Could you check a few things on this model? Use its own coordinates, in mm. A direction names the side the tool comes from. Round coordinates to 2 decimals unless told otherwise and drop trailing zeros. Order: outer loops, then holes, each group sorted by start corner. A loop starts at its lowest first (then second) coordinate and runs counter-clockwise, first axis right, second up. Notation, with made-up numbers: (-12.75, 38) - (24.25, 38) arc R25 cw to (24.25, 70) - close; hole circle Ø4 at (72, 78). An arc over 180 degrees is marked (long way). Use one line per item in the form item = value.
from build123d import *

# Parameters (mm, degrees)
BOSS_EXTRU_1_DEPTH                  = 3.175
ESQUISSE3_W                         = 42
ESQUISSE3_H                         = 16
BOSS_EXTRU_2_DEPTH                  = 45
ESQUISSE4_W                         = 20
ESQUISSE4_H                         = 16
ENL_V_MAT_EXTRU_1_DEPTH             = 123.60232716
ESQUISSE5_W                         = 22
ESQUISSE5_H                         = 31.825
ENL_V_MAT_EXTRU_2_DEPTH             = 128.730184373
CONG_1_R                            = 5
D_GAGEMENT_M3_51_D                  = 3.9
D_GAGEMENT_M31_D                    = 3.4
ESQUISSE11_R                        = 17.225
ENL_V_MAT_EXTRU_3_DEPTH             = 123.60232716
DIAM_TRE_DU_PER_AGE_4_5_4_5_2_D     = 4.5
DIAM_TRE_DU_PER_AGE_4_5_4_5_2_DEPTH = 5.8
ENL_V_MAT_EXTRU_4_DEPTH             = 18


with BuildPart() as part:
    # Esquisse1 → Boss.-Extru.1 (new, symmetric)
    with BuildSketch(Plane(origin=(0, 0, 0), x_dir=(1, 0, 0), z_dir=(0, 1, 0))):
        with BuildLine():
            Line((-40, 59), (40, 59))
            ThreePointArc((40, 59), (99, 0), (40, -59))
            Line((40, -59), (-40, -59))
            ThreePointArc((-40, -59), (-99, 0), (-40, 59))
        make_face()
    extrude(amount=BOSS_EXTRU_1_DEPTH, both=True)

    # Esquisse3 → Boss.-Extru.2 (add)
    with BuildSketch(Plane(origin=(0, 0, 0), x_dir=(1, 0, 0), z_dir=(0, 1, 0))):
        with Locations((-62.5, 0)):
            Rectangle(ESQUISSE3_W, ESQUISSE3_H)
    extrude(amount=BOSS_EXTRU_2_DEPTH)

    # Esquisse4 → Enlèv. mat.-Extru.1 (cut, through all)
    with BuildSketch(Plane(origin=(0, 3.175, 0), x_dir=(1, 0, 0), z_dir=(0, 1, 0))):
        with Locations((-31.5, 0)):
            Rectangle(ESQUISSE4_W, ESQUISSE4_H)
    extrude(amount=-ENL_V_MAT_EXTRU_1_DEPTH, mode=Mode.SUBTRACT)

    # Esquisse5 → Enlèv. mat.-Extru.2 (cut, through all)
    with BuildSketch(Plane.XY.offset(8)):
        with Locations((-72.5, 29.0875)):
            Rectangle(ESQUISSE5_W, ESQUISSE5_H)
    extrude(amount=-ENL_V_MAT_EXTRU_2_DEPTH, mode=Mode.SUBTRACT)

    # Congé1
    cong_1_edges = [part.edges().sort_by_distance(p)[0] for p in [
        (-72.5, 13.175, -8),
        (-61.5, 13.175, 0),
        (-83.5, 13.175, 0),
        (-61.5, 29.0875, 8),
        (-61.5, 29.0875, -8),
        (-72.5, 13.175, 8),
    ]]
    fillet(cong_1_edges, radius=CONG_1_R)

    # Dégagement M3.51 (through all)
    with Locations(Plane(origin=(-41.5, 0, 0), x_dir=(0, 0, -1), z_dir=(1, 0, 0))):
        with Locations((0, 32.55)):
            Hole(D_GAGEMENT_M3_51_D / 2)

    # Dégagement M31 (through all)
    with Locations(Plane(origin=(0, 3.175, 0), x_dir=(1, 0, 0), z_dir=(0, 1, 0))):
        with Locations((60.016012145, -11.55625), (40, 23.1125), (19.983987855, -11.55625)):
            Hole(D_GAGEMENT_M31_D / 2)

    # Esquisse11 → Enlèv. mat.-Extru.3 (cut, through all)
    with BuildSketch(Plane(origin=(0, 3.175, 0), x_dir=(1, 0, 0), z_dir=(0, 1, 0))):
        with Locations(Location((40, 0, 0), (0, 0, 270))):
            Circle(ESQUISSE11_R)
    extrude(amount=-ENL_V_MAT_EXTRU_3_DEPTH, mode=Mode.SUBTRACT)

    # Diamètre du perçage Ø4.5 (4.5)2
    with Locations(Plane(origin=(0, -3.175, 0), x_dir=(-1, 0, 0), z_dir=(0, -1, 0))):
        with Locations((78.5, 0), (66.5, 0)):
            Hole(DIAM_TRE_DU_PER_AGE_4_5_4_5_2_D / 2, depth=DIAM_TRE_DU_PER_AGE_4_5_4_5_2_DEPTH)

    # Esquisse14 → Enlèv. mat.-Extru.4 (cut)
    with BuildSketch(Plane.ZY.offset(61.5)):
        Polygon((4.67653718, 32.55), (2.33826859, 36.6), (-2.33826859, 36.6), (-4.67653718, 32.55), (-2.33826859, 28.5), (2.33826859, 28.5), align=None)
    extrude(amount=-ENL_V_MAT_EXTRU_4_DEPTH, mode=Mode.SUBTRACT)


solid = part.part
Item 1: If we mould it in two halves opening along Z, with no side actions, what happens to faces 4 (the face through (-1, 0, -59)), 5 (the face through (-98.986, 0.044, 1.297)), 6 (the face through (-43.5, 34.4, 1)), 7 (the face through (-73, 13.175, 0))? For each: released by +Z, released by -Z, zero draft, split by the parting line, or undercut.
Found:
face_4 = released by -Z
face_5 = split by the parting line
face_6 = undercut
face_7 = zero draft
Item 2: I need wall thicknesses on L1, parallel to Y at x = -42.3, z = 0 (3 decimals); L2, parallel to X at y = 0, z = 10 (3 decimals); L3, parallel to Y at x = 11, z = 42.5 (3 decimals). Which ranges of each line are inside material? Lowest first, please.
Found:
L1 = -3.175 to 30.6, 34.5 to 45
L2 = -98.146 to 19.3, 20.668 to 25.975, 54.025 to 59.332, 60.7 to 98.146
L3 = -3.175 to 3.175
Item 3: Imagine slicing it at D-D on x = 5.5. Please give me the cut outline in (y, z) (3 decimals), plus the area to 3 significant figures.
Found:
outline = (-3.175, -59) - (3.175, -59) - (3.175, 59) - (-3.175, 59) - close
area = 749 mm2
Item 4: Will these pins go through, and if not, where does the flat tip stop? P1, Ø5, axis at x = -70, z = -1.5, coming from the +Y side (3 decimals); P2, Ø3, axis at y = 3.5, z = -33, coming from the +X side; P3, Ø10, axis at x = 31.5, z = 11.5, coming from the +Y side (3 decimals); P4, Ø5, axis at x = -66.5, z = 0, coming from the -Y side (3 decimals).
Found:
P1 = 13.175
P2 = 89.86
P3 = 3.175
P4 = -3.175
Item 5: Imagine slicing it at A-A on z = 0. State how many separate pieces and enclosed holes the cut face has, plus the area to 3 significant figures.
Found:
separate_pieces = 4
enclosed_holes = 0
area = 1,760 mm2
Item 6: Imagine slicing it at B-B on z = -13.5. Please give me the cut outline in (x, y) (3 decimals).
Found:
outline = (-97.435, -3.175) - (29.302, -3.175) - (29.302, 3.175) - (-97.435, 3.175) - close; (50.698, -3.175) - (97.435, -3.175) - (97.435, 3.175) - (50.698, 3.175) - close
Item 7: For faces 1 (the face through (-68.748, -0.234, -0.099)), 2 (the face through (-61.5, 41, 0)), 3 (the face through (-53, 19, -8)), which set-ups out of +Z, -Z, +X, -X, +Y, -Y let a thin tool reach every point of the face, with its end or its side?
Found:
face_1 = -Y
face_2 = +Z, -Z, -X, +Y
face_3 = -Z, +X, -X, +Y
